Can you work these out from the model? Positions are in its coordinate system, mm. A direction names the side the tool comes from. Round coordinates to 2 decimals unless told otherwise and drop trailing zeros. Write each loop counter-clockwise with the first axis right and the second up, starting at its lowest first coordinate (ties: lowest second). Pieces come first, ordered by that corner, then holes. Notation, with made-up numbers: (3.25, 46.25) -> (11.25, 46.25) arc R14 ccw to (11.25, 66.25) -> close; hole circle Ø1 at (0, 74.25). An arc over 180 degrees is marked (long way). Use CSV: the item, a comma, the result in double quotes.
Autodesk Inventor part; units mm, degrees
ref_plane "YZ Plane" through (0, 0, 0) normal (1, 0, 0) x (0, 1, 0)
ref_plane "XZ Plane" through (0, 0, 0) normal (0, 1, 0) x (-1, 0, 0)
ref_plane "XY Plane" through (0, 0, 0) normal (0, 0, 1) x (1, 0, 0)
sketch "草图1" plane through (0, 0, 0) normal (1, 0, 0) x (0, 1, 0)
  line L0 (-600, 900) -> (600, 900)
  line L1 (600, 900) -> (600, -900)
  line L2 (600, -900) -> (-600, -900)
  line L3 (-600, -900) -> (-600, 900)
  line L4 (-600, 900) -> (600, -900) construction
  line L5 (600, 900) -> (-600, -900) construction
  point P0 (0, 0)
  dimension "d0" = 1200
  dimension "d1" = 1800
extrude "拉伸1" add sketch "草图1" along normal blind 500
sketch "草图2" plane through (500, 0, 0) normal (1, 0, 0) x (0, 0, -1)
  line L0 (-900, 600) -> (-900, -600)
  line L1 (-900, 600) -> (-850, 600)
  line L2 (900, -600) -> (900, 600)
  line L3 (-850, 600) -> (-850, -600)
  line L4 (-900, -600) -> (-900, -550)
  line L5 (-900, -550) -> (900, -550)
  line L6 (-900, 600) -> (-900, 550)
  line L7 (-900, 550) -> (900, 550)
  line L8 (900, 600) -> (-900, 600)
  line L9 (900, 600) -> (850, 600)
  line L10 (850, 600) -> (850, -600)
  line L11 (-900, -600) -> (900, -600)
  line L12 (-850, 0) -> (-850, -25)
  line L13 (-850, -25) -> (-850, 25)
  line L14 (-850, 25) -> (850, 25)
  line L15 (850, -25) -> (-850, -25)
  point P0 (0, 0)
  point P1 (-850, -550)
  point P2 (850, -550)
  point P3 (850, 550)
  point P4 (-850, 550)
  dimension "d10" = 50
  dimension "d11" = 50
  dimension "d12" = 50
  dimension "d13" = 50
  dimension "d14" = 25
  dimension "d15" = 50
extrude "拉伸2" cut sketch "草图2" against normal blind 450 contours L7 L10 L14 L3 | L3 L15 L10 L5
properties part number "书架" material "木材(枫木)"
Q1. Suppose I cut it at A-A (x = 258.5). Write out the boundary of the cut face in (y, z), and give its area (3 significant figures).
Resolved:
outline,"(-600, -900) -> (600, -900) -> (600, 900) -> (-600, 900) -> close; hole (-550, -850) -> (-25, -850) -> (-25, 850) -> (-550, 850) -> close; hole (25, -850) -> (550, -850) -> (550, 850) -> (25, 850) -> close"
area,"375,000 mm^2"
Q2. Please list where these lines run through material, in increasing order: probe 1 along Y at (x, z) = (100, -46); probe 2 along Z at (x, y) = (114, -264); probe 3 along X at (y, z) = (-42, -299).
Resolved:
probe 1,"y = -600 to -550, -25 to 25, 550 to 600"
probe 2,"z = -900 to -850, 850 to 900"
probe 3,"x = 0 to 50"
Q3. On a 3-axis mill with a long thin cutter (end or side, diameter ignored), from which of +Z, -Z, +X, -X, +Y, -Y can I reach the whole of each face in a straight line? I mean faces 1 (the face through (500, -3, 4)), 2 (the face through (278, 291, 850)). Say none if no direction works.
Resolved:
face 1,"+Z, -Z, +X, +Y, -Y"
face 2,"+X"
Q4. Suppose I cut it at C-C (y = -360). Write out the boundary of the cut face in (x, z).
Resolved:
outline,"(0, -900) -> (500, -900) -> (500, -850) -> (50, -850) -> (50, 850) -> (500, 850) -> (500, 900) -> (0, 900) -> close"
Q5. Will this pin go through, and if not, where does the flat tip stop? P1, Ø1.5, axis at y = -40.5, z = -523, coming from the +X side.
Resolved:
P1,"stops at x = 50"
Q6. If we mould it in two halves opening along Z, with no side actions, what happens to faces 3 (the face through (246, 8, -900)), 4 (the face through (246, 600, 13)), 5 (the face through (278, -25, -12))? For each: released by +Z, released by -Z, zero draft, split by the parting line, or undercut.
Resolved:
face 3,"released by -Z"
face 4,"zero draft"
face 5,"undercut"
Q7. Suppose I cut it at B-B (z = 146). Write out the boundary of the cut face in (x, y), and give its area (4 significant figures).
Resolved:
outline,"(0, -600) -> (500, -600) -> (500, -550) -> (50, -550) -> (50, -25) -> (500, -25) -> (500, 25) -> (50, 25) -> (50, 550) -> (500, 550) -> (500, 600) -> (0, 600) -> close"
area,"127,500 mm^2"
